Input: dimensioned drawing with shaded views. Units: mm. Origin: part minimum x, y, z. Give positions to 0.01 mm unless a question says otherwise; leave off trailing zeros. Order: outer loops, then holes, each group sorted by start corner. A loop starts at its lowest first (then second) coordinate and runs counter-clockwise, first axis right, second up. Notation, with made-up numbers: (75.5, -2.75) -> (93.5, -2.75) arc R25 cw to (93.5, 36.25) -> close; hole circle Ø9 at (31, 40.25). An arc over 180 degrees is marked (long way). One line per question, with ' | ' between items. Start each with the question number.
(1) First-contact query: pin 1 Ø3.5 at (x, y) = (25, 10) entering from -Z. Flat tip, straight axial feed; report the tip coordinate or a pass-through.
(2) Section D-D (x = 26). Return loops of the section in (y, z).
(3) Mould query, pull axis Y, two halves, no side actions, for the marked faces 1, 2 and 3. Classes: +Y half, -Y half, draft (parallel to the pull), parting line (faces both ways), or undercut.
(4) Ray query, L1, parallel to Y at x = 3, z = 1.65; L2, parallel to Y at x = 25, z = 0.95; L3, parallel to Y at x = 4, z = 1.35. Return the intervals inside material, ascending.
(5) Section C-C (z = 0.6). Return loops of the section in (x, y).
(6) Section A-A (x = 3). Return loops of the section in (y, z).
(7) Section B-B (y = 10). Return loops of the section in (x, z), then the cut area to 3 significant figures.
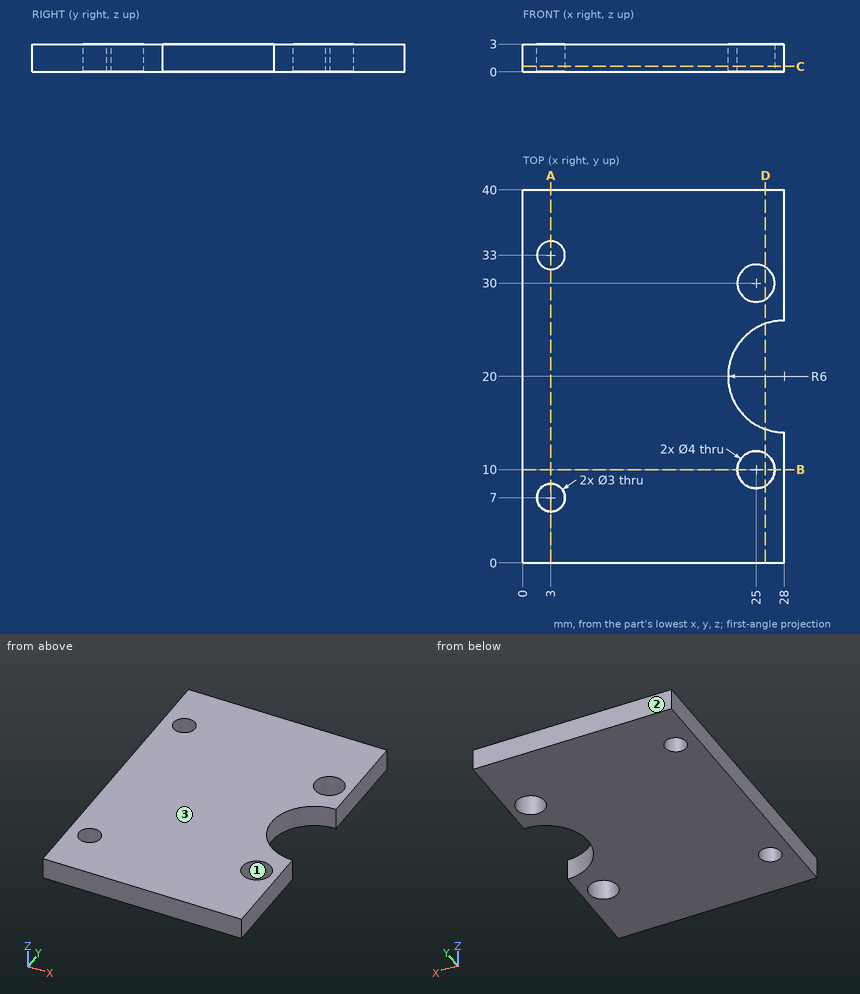
Response:
1) pin 1: passes through
2) outline: (0, 0) -> (8.27, 0) -> (8.27, 3) -> (0, 3) -> close; (11.73, 0) -> (14.34, 0) -> (14.34, 3) -> (11.73, 3) -> close; (25.66, 0) -> (28.27, 0) -> (28.27, 3) -> (25.66, 3) -> close; (31.73, 0) -> (40, 0) -> (40, 3) -> (31.73, 3) -> close
3) face 1: undercut | face 2: +Y half | face 3: draft
4) L1: y = 0 to 5.5, 8.5 to 31.5, 34.5 to 40 | L2: y = 0 to 8, 12 to 14.8, 25.2 to 28, 32 to 40 | L3: y = 0 to 5.88, 8.12 to 31.88, 34.12 to 40
5) outline: (0, 0) -> (28, 0) -> (28, 14) arc R6 cw to (28, 26) -> (28, 40) -> (0, 40) -> close; hole circle Ø3 at (3, 7); hole circle Ø3 at (3, 33); hole circle Ø4 at (25, 10); hole circle Ø4 at (25, 30)
6) outline: (0, 0) -> (5.5, 0) -> (5.5, 3) -> (0, 3) -> close; (8.5, 0) -> (31.5, 0) -> (31.5, 3) -> (8.5, 3) -> close; (34.5, 0) -> (40, 0) -> (40, 3) -> (34.5, 3) -> close
7) outline: (0, 0) -> (23, 0) -> (23, 3) -> (0, 3) -> close; (27, 0) -> (28, 0) -> (28, 3) -> (27, 3) -> close | area: 72.0 mm^2
